from build123d import *

# Parameters (mm, degrees)
CHAMFER1_SIZE      = 0.5
CHAMFER2_SIZE      = 0.3
CUT_EXTRUDE1_DEPTH = 2.5
CHAMFER3_SIZE      = 0.3


with BuildPart() as part:
    # Sketch1 → Revolve1 (revolve)
    with BuildSketch(Plane.XY):
        Polygon((0, 0), (0, 2.75), (3, 2.75), (3, 1.49), (19, 1.49), (19, 0), align=None)
    revolve(axis=Axis((-88.705490849, 0, 0), (1, 0, 0)))

    # Chamfer1
    chamfer1_edges = [part.edges().sort_by_distance(p)[0] for p in [
        (19, -1.49, 0),
    ]]
    chamfer(chamfer1_edges, length=CHAMFER1_SIZE)

    # Chamfer2
    chamfer2_edges = [part.edges().sort_by_distance(p)[0] for p in [
        (0, -2.75, 0),
    ]]
    chamfer(chamfer2_edges, length=CHAMFER2_SIZE)

    # Sketch3 → Cut-Extrude1 (cut)
    with BuildSketch(Plane(origin=(0, 0, 0), x_dir=(0, 0, -1), z_dir=(1, 0, 0))):
        Polygon((-1.443375673, 0), (-0.721687836, -1.25), (0.721687836, -1.25), (1.443375673, 0), (0.721687836, 1.25), (-0.721687836, 1.25), align=None)
    extrude(amount=CUT_EXTRUDE1_DEPTH, mode=Mode.SUBTRACT)

    # Chamfer3
    chamfer3_edges = [part.edges().sort_by_distance(p)[0] for p in [
        (0, 0.625, 1.082531755),
        (0, -0.625, 1.082531755),
        (0, -1.25, 0),
        (0, -0.625, -1.082531755),
        (0, 0.625, -1.082531755),
        (0, 1.25, 0),
    ]]
    chamfer(chamfer3_edges, length=CHAMFER3_SIZE)


solid = part.part
CAD build for the part. Positions are in the model's coordinates, mm. A direction names the side the tool comes from. Round coordinates to 2 decimals unless told otherwise and drop trailing zeros. Order: outer loops, then holes, each group sorted by start corner. A loop starts at its lowest first (then second) coordinate and runs counter-clockwise, first axis right, second up. Notation, with made-up numbers: (-33, 8.5) -> (-7, 8.5) arc R22 ccw to (-7, 26.5) -> close; hole circle Ø1 at (58.25, 4.5). An arc over 180 degrees is marked (long way). Write each question's results on one line, items separated by ' | '.
1. 3-axis set-ups, long thin cutter, end or side, ignore diameter. For faces 1 (the face through (0.15, -0.69, 1.22)), 2 (the face through (19, 0, 0)), 3 (the face through (10.858, -0.194, 1.477)): which of +Z, -Z, +X, -X, +Y, -Y reach the whole face in a straight line?
Findings below:
face 1: -X | face 2: +Z, -Z, +X, +Y, -Y | face 3: +X
2. Cut at A-A (z = 0). Give the cut face in (x, y), plus the area to 3 significant figures.
Findings below:
outline: (0, -2.45) -> (0.3, -2.75) -> (3, -2.75) -> (3, -1.49) -> (18.5, -1.49) -> (19, -0.99) -> (19, 0.99) -> (18.5, 1.49) -> (3, 1.49) -> (3, 2.75) -> (0.3, 2.75) -> (0, 2.45) -> (0, 1.55) -> (0.3, 1.25) -> (2.5, 1.25) -> (2.5, -1.25) -> (0.3, -1.25) -> (0, -1.55) -> close | area: 57.5 mm²
3. Pull direction Y, two halves, no side cores. Call faces 4 (the face through (1, 1.25, 0)), 5 (the face through (1.669, -0.596, -2.685)), 6 (the face through (3, 1.2, -1.2)): pulls with the +Y half, pulls with the -Y half, needs draft (parallel to the pull), parting line crosses it, or undercut.
Findings below:
face 4: undercut | face 5: parting line crosses it | face 6: needs draft
4. Wall check: line 1 along Y through (x, z) = (13.25, 0.05); line 2 along X through (y, z) = (2, 0.45); line 3 along Y through (x, z) = (6.5, -0.35). Give the ranges that are in metal, low to high. Write a range as [from, to].
Findings below:
line 1: y = [-1.49, 1.49] | line 2: x = [0, 3] | line 3: y = [-1.45, 1.45]
5. Cut at B-B (x = 14.25). Give the cut face in (y, z), plus the area to 3 significant figures.
Findings below:
outline: circle Ø2.98 at (0, 0) | area: 6.97 mm²
6. Flat gauge pin, fed straight in: P1, Ø3, axis at x = 7.5, y = -2, coming from the -Z side. Where does the tip first touch, or does it go through?
Findings below:
P1: stops at z = -1.4
